```python
from build123d import *

# Parameters (mm, degrees)
BOSS_EXTRUDE1_DEPTH = 15
SKETCH2_R           = 2.25
BOSS_EXTRUDE2_DEPTH = 15
CHAMFER4_SIZE       = 0.5
CHAMFER5_SIZE       = 0.5
SKETCH4_R           = 3
CUT_EXTRUDE1_DEPTH  = 5


with BuildPart() as part:
    # Sketch1 → Boss-Extrude1 (new body)
    with BuildSketch(Plane.XY):
        Polygon((-21.283297093, 0), (8.716702907, 0), (8.716702907, -19.069471621), (-1.283297093, -39.344386688), (-11.283297093, -39.344386688), (-21.283297093, -19.069471621), align=None)
    extrude(amount=BOSS_EXTRUDE1_DEPTH)

    # Sketch2 → Boss-Extrude2 (add)
    with BuildSketch(Plane(origin=(0, 0, 0), x_dir=(1, 0, 0), z_dir=(0, 1, 0))):
        with Locations((-16.283297093, -7.5)):
            Circle(SKETCH2_R)
        with Locations((3.716702907, -7.5)):
            Circle(SKETCH2_R)
    extrude(amount=BOSS_EXTRUDE2_DEPTH)

    # Chamfer4
    chamfer4_edges = [part.edges().sort_by_distance(p)[0] for p in [
        (-18.533297093, 15, 7.5),
    ]]
    chamfer(chamfer4_edges, length=CHAMFER4_SIZE)

    # Chamfer5
    chamfer5_edges = [part.edges().sort_by_distance(p)[0] for p in [
        (1.466702907, 15, 7.5),
    ]]
    chamfer(chamfer5_edges, length=CHAMFER5_SIZE)

    # Sketch4 → Cut-Extrude1 (cut)
    with BuildSketch(Plane(origin=(0, -39.344386688, 0), x_dir=(-1, 0, 0), z_dir=(0, -1, 0))):
        with Locations((6.283297093, -7.5)):
            Circle(SKETCH4_R)
    extrude(amount=-CUT_EXTRUDE1_DEPTH, mode=Mode.SUBTRACT)


solid = part.part
```
For this review, take the finished solid that the model builds, in its own axes (mm). A direction names the side the tool comes from. Give positions to 0.01 mm unless a question says otherwise; leave off trailing zeros. Write each loop counter-clockwise with the first axis right and the second up, starting at its lowest first coordinate (ties: lowest second). Pieces come first, ordered by that corner, then holes. Notation, with made-up numbers: M -7,-1 L 47,-1 A23 cw 47,24 Z; hole C 66.5,23 d10. An arc over 180 degrees is marked long. One line per item, written item: value.
1) For faces 1 (the flat face through (-16, 15, 7)), 2 (the cylindrical face through (-9.145, -36.879, 6.599)), 3 (the cylindrical face through (-14.14, 7.15, 6.82)), list the 3-axis set-ups (+Z, -Z, +X, -X, +Y, -Y) from which the entire face can be reached by the end or side of a thin tool; tool diameter is ignored.
Results are:
face 1: +Z, -Z, +X, -X, +Y
face 2: -Y
face 3: +Y
2) The part is to be moulded in two halves that separate along X. For faces 4 (the flat face through (4, 15, 7)), 5 (the flat face through (-16.213, -29.349, 7.395)), 6 (the cylindrical face through (3.42, 7.15, 5.27)), 7 (the flat face through (-6, -34.344, 7)), say which applies: +X half, -X half, draft (parallel to the pull), parting line (faces both ways), or undercut.
Results are:
face 4: draft
face 5: -X half
face 6: undercut
face 7: undercut
3) For P1, Ø2, axis at x = 2.5, y = 2.5, coming from the +Z side; P2, Ø5, axis at x = -5.5, z = 8.5, coming from the -Y side; P3, Ø1.8, axis at x = -7.5, z = 8.5, coming from the -Y side; P4, Ø3, axis at x = 0.5, y = 2.5, coming from the -Z side, all flat-tipped, find the tip position at first contact; note any pin that passes through.
Results are:
P1: stops at z = 9.74
P2: stops at y = -39.34
P3: stops at y = -34.34
P4: stops at z = 6.05
4) For line 1 (Y direction, x = -2, z = 2); line 2 (X direction, y = -36.1, z = 7.5); line 3 (X direction, y = 8, z = 8.25), list the stretches that pass through material, from the lowest coordinate up. Write a range as from..to.
Results are:
line 1: y = -39.34..0
line 2: x = -12.88..-9.28, -3.28..0.32
line 3: x = -18.4..-14.16, 1.6..5.84
5) Take a section at B-B, the plane y = 7. Write out the cut boundary in (x, z).
Results are:
outline: C -16.28,7.5 d4.5; C 3.72,7.5 d4.5
6) Take a section at C-C, the plane x = 6.5. Write out the cut boundary in (y, z).
Results are:
outline: M -23.56,0 L 0,0 L 0,15 L -23.56,15 Z
7) Take a section at A-A, the plane z = 13. Write out the cut boundary in (x, y).
Results are:
outline: M -21.28,-19.07 L -11.28,-39.34 L -1.28,-39.34 L 8.72,-19.07 L 8.72,0 L -21.28,0 Z
8) Take a section at D-D, the plane z = 7.5. Write out the cut boundary in (x, y), then the cut area to 3 significant figures.
Results are:
outline: M -21.28,-19.07 L -11.28,-39.34 L -9.28,-39.34 L -9.28,-34.34 L -3.28,-34.34 L -3.28,-39.34 L -1.28,-39.34 L 8.72,-19.07 L 8.72,0 L 5.97,0 L 5.97,14.5 L 5.47,15 L 1.97,15 L 1.47,14.5 L 1.47,0 L -14.03,0 L -14.03,14.5 L -14.53,15 L -18.03,15 L -18.53,14.5 L -18.53,0 L -21.28,0 Z
area: 1,080 mm²
